Read the model definition and answer for the solid it produces. Units are mm, in the model's axes. Face numbers are marked on the shaded views. Give positions to 0.01 mm unless a question says otherwise; leave off trailing zeros. Write each loop counter-clockwise with the first axis right and the second up, starting at its lowest first coordinate (ties: lowest second). Pieces come first, ordered by that corner, then holes. Notation, with made-up numbers: M 74.25,31.5 L 120.25,31.5 A13 cw 120.25,56.5 Z; hole C 45,5 d4. An arc over 180 degrees is marked long. Put each result on its own line as item: value.
Autodesk Inventor part; units mm, degrees
ref_plane "YZ Plane" through (0, 0, 0) normal (1, 0, 0) x (0, 1, 0)
ref_plane "XZ Plane" through (0, 0, 0) normal (0, 1, 0) x (-1, 0, 0)
ref_plane "XY Plane" through (0, 0, 0) normal (0, 0, 1) x (1, 0, 0)
sketch "Sketch1" plane through (0, 0, 0) normal (0, 0, 1) x (1, 0, 0)
  circle A0 centre (-2.41, 40.64) radius 12.5
  line L0 (-16.506, 28.736) -> (-19.006, 26.236)
  arc A1 (-14.314, 26.544) -> (-16.506, 28.736) centre (-15.41, 27.64) ccw
  line L1 (-16.814, 24.044) -> (-14.314, 26.544)
  arc A2 (-19.006, 26.236) -> (-16.814, 24.044) centre (-17.91, 25.14) ccw
  line L2 (-19.006, 55.044) -> (-16.506, 52.544)
  arc A3 (-16.506, 52.544) -> (-14.314, 54.736) centre (-15.41, 53.64) ccw
  line L3 (-14.314, 54.736) -> (-16.814, 57.236)
  arc A4 (-16.814, 57.236) -> (-19.006, 55.044) centre (-17.91, 56.14) ccw
  line L4 (9.494, 26.544) -> (11.994, 24.044)
  arc A5 (11.686, 28.736) -> (9.494, 26.544) centre (10.59, 27.64) ccw
  line L5 (14.186, 26.236) -> (11.686, 28.736)
  arc A6 (11.994, 24.044) -> (14.186, 26.236) centre (13.09, 25.14) ccw
  line L6 (11.686, 52.544) -> (14.186, 55.044)
  arc A7 (9.494, 54.736) -> (11.686, 52.544) centre (10.59, 53.64) ccw
  line L7 (11.994, 57.236) -> (9.494, 54.736)
  arc A8 (14.186, 55.044) -> (11.994, 57.236) centre (13.09, 56.14) ccw
  circle A9 centre (20.14, 70.64) radius 2.5
  circle A10 centre (20.14, 10.64) radius 2.5
  circle A11 centre (100.14, 40.64) radius 3.57
  line L8 (-22.41, 20.64) -> (-22.41, 60.64)
  line L9 (-22.41, 60.64) -> (17.59, 80.64)
  line L10 (17.59, 80.64) -> (117.59, 80.64)
  line L11 (117.59, 80.64) -> (117.59, 0.64)
  line L12 (117.59, 0.64) -> (20.14, 0.64)
  line L13 (20.14, 0.64) -> (-22.41, 20.64)
  point P0 (0, 0)
  dimension "d0" = 20
  dimension "d1" = 0
  dimension "d2" = 80
  dimension "d3" = 90
  dimension "d4" = 90
  dimension "d5" = 10
  dimension "d6" = 100
  dimension "d7" = 140
  dimension "d8" = 40
  dimension "d9" = 20
extrude "Extrusion1" add sketch "Sketch1" along normal blind 3
fillet "Fillet1" radius 5 6 edges at (117.59, 80.64, 1.5) (117.59, 0.64, 1.5) (17.59, 80.64, 1.5) (-22.41, 60.64, 1.5) (-22.41, 20.64, 1.5) (20.14, 0.64, 1.5)
sketch "Sketch2" plane through (0, 0, 0) normal (0, 0, -1) x (-1, 0, 0)
  circle A0 centre (2.41, 40.64) radius 12.5
  circle A1 centre (-100.14, 40.64) radius 3.57
  circle A2 centre (-20.14, 10.64) radius 2.5
  circle A3 centre (-20.14, 70.64) radius 2.5
  arc A4 (-11.686, 52.544) -> (-9.494, 54.736) centre (-10.59, 53.64) ccw
  line L0 (-11.686, 52.544) -> (-14.186, 55.044)
  arc A5 (-11.994, 57.236) -> (-14.186, 55.044) centre (-13.09, 56.14) ccw
  line L1 (-11.994, 57.236) -> (-9.494, 54.736)
  arc A6 (-9.494, 26.544) -> (-11.686, 28.736) centre (-10.59, 27.64) ccw
  line L2 (-9.494, 26.544) -> (-11.994, 24.044)
  arc A7 (-14.186, 26.236) -> (-11.994, 24.044) centre (-13.09, 25.14) ccw
  line L3 (-14.186, 26.236) -> (-11.686, 28.736)
  arc A8 (19.006, 55.044) -> (16.814, 57.236) centre (17.91, 56.14) ccw
  line L4 (19.006, 55.044) -> (16.506, 52.544)
  arc A9 (14.314, 54.736) -> (16.506, 52.544) centre (15.41, 53.64) ccw
  line L5 (14.314, 54.736) -> (16.814, 57.236)
  arc A10 (16.506, 28.736) -> (14.314, 26.544) centre (15.41, 27.64) ccw
  line L6 (16.506, 28.736) -> (19.006, 26.236)
  arc A11 (16.814, 24.044) -> (19.006, 26.236) centre (17.91, 25.14) ccw
  line L7 (16.814, 24.044) -> (14.314, 26.544)
  arc A12 (-21.2565, 0.64) -> (-19.1296, 1.1149) centre (-21.2565, 5.64) ccw
  line L8 (-19.1296, 1.1149) -> (19.5369, 19.2896)
  arc A13 (19.5369, 19.2896) -> (22.41, 23.8146) centre (17.41, 23.8146) ccw
  line L9 (22.41, 23.8146) -> (22.41, 57.5498)
  arc A14 (22.41, 57.5498) -> (19.6461, 62.022) centre (17.41, 57.5498) ccw
  line L10 (19.6461, 62.022) -> (-16.5343, 80.1121)
  arc A15 (-16.5343, 80.1121) -> (-18.7703, 80.64) centre (-18.7703, 75.64) ccw
  line L11 (-18.7703, 80.64) -> (-112.59, 80.64)
  arc A16 (-112.59, 80.64) -> (-117.59, 75.64) centre (-112.59, 75.64) ccw
  line L12 (-117.59, 75.64) -> (-117.59, 5.64)
  arc A17 (-117.59, 5.64) -> (-112.59, 0.64) centre (-112.59, 5.64) ccw
  line L13 (-112.59, 0.64) -> (-21.2565, 0.64)
  point P0 (0, 0)
hole "Hole1" at (100.14, 40.64, 0) direction (0, 0, 1) diameter 12 depth 1
sketch "Sketch3" plane through (0, 0, 0) normal (0, 0, -1) x (-1, 0, 0)
  circle A0 centre (-20.14, 10.64) radius 2.5
  circle A1 centre (-100.14, 40.64) radius 6
  circle A2 centre (2.41, 40.64) radius 12.5
  circle A3 centre (-20.14, 10.64) radius 2.5
  circle A4 centre (-20.14, 70.64) radius 2.5
  arc A5 (-11.686, 52.544) -> (-9.494, 54.736) centre (-10.59, 53.64) ccw
  line L0 (-11.686, 52.544) -> (-14.186, 55.044)
  arc A6 (-11.994, 57.236) -> (-14.186, 55.044) centre (-13.09, 56.14) ccw
  line L1 (-11.994, 57.236) -> (-9.494, 54.736)
  arc A7 (-9.494, 26.544) -> (-11.686, 28.736) centre (-10.59, 27.64) ccw
  line L2 (-9.494, 26.544) -> (-11.994, 24.044)
  arc A8 (-14.186, 26.236) -> (-11.994, 24.044) centre (-13.09, 25.14) ccw
  line L3 (-14.186, 26.236) -> (-11.686, 28.736)
  arc A9 (19.006, 55.044) -> (16.814, 57.236) centre (17.91, 56.14) ccw
  line L4 (19.006, 55.044) -> (16.506, 52.544)
  arc A10 (14.314, 54.736) -> (16.506, 52.544) centre (15.41, 53.64) ccw
  line L5 (14.314, 54.736) -> (16.814, 57.236)
  arc A11 (16.506, 28.736) -> (14.314, 26.544) centre (15.41, 27.64) ccw
  line L6 (16.506, 28.736) -> (19.006, 26.236)
  arc A12 (16.814, 24.044) -> (19.006, 26.236) centre (17.91, 25.14) ccw
  line L7 (16.814, 24.044) -> (14.314, 26.544)
  arc A13 (-21.2565, 0.64) -> (-19.1296, 1.1149) centre (-21.2565, 5.64) ccw
  line L8 (-19.1296, 1.1149) -> (19.5369, 19.2896)
  arc A14 (19.5369, 19.2896) -> (22.41, 23.8146) centre (17.41, 23.8146) ccw
  line L9 (22.41, 23.8146) -> (22.41, 57.5498)
  arc A15 (22.41, 57.5498) -> (19.6461, 62.022) centre (17.41, 57.5498) ccw
  line L10 (19.6461, 62.022) -> (-16.5343, 80.1121)
  arc A16 (-16.5343, 80.1121) -> (-18.7703, 80.64) centre (-18.7703, 75.64) ccw
  line L11 (-18.7703, 80.64) -> (-112.59, 80.64)
  arc A17 (-112.59, 80.64) -> (-117.59, 75.64) centre (-112.59, 75.64) ccw
  line L12 (-117.59, 75.64) -> (-117.59, 5.64)
  arc A18 (-117.59, 5.64) -> (-112.59, 0.64) centre (-112.59, 5.64) ccw
  line L13 (-112.59, 0.64) -> (-21.2565, 0.64)
  circle A19 centre (-20.14, 70.64) radius 2.0572
  circle A20 centre (-20.14, 10.64) radius 2.0572
  point P0 (0, 0)
hole "Hole2" at (20.14, 10.64, 0) at (20.14, 70.64, 0) direction (0, 0, 1) diameter 8.1 depth 1
properties part number "Y Slider" material "Aluminum 6061"
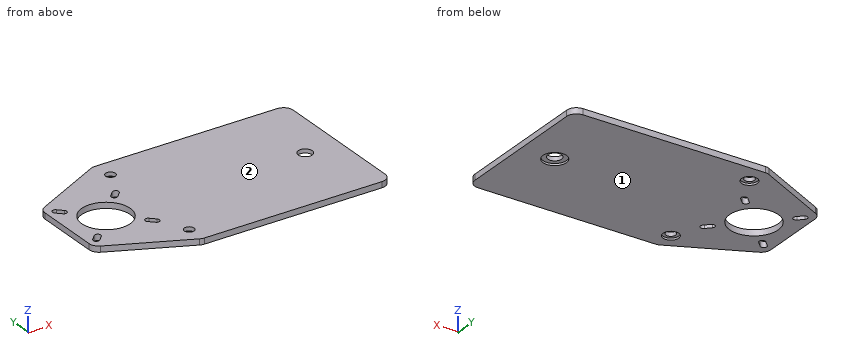
(1) Section B-B on z = 1.8 is taken. Give the number of separate pieces and of enclosed holes in the cut face, and give its area (3 significant figures).
Result:
separate pieces: 1
enclosed holes: 8
area: 9,720 mm²
(2) Section C-C on y = 40.64 is taken. Determine the outline of the cut face in (x, z).
Result:
outline: M -22.41,0 L -14.91,0 L -14.91,3 L -22.41,3 Z; M 10.09,0 L 94.14,0 L 94.14,1 L 96.57,1 L 96.57,3 L 10.09,3 Z; M 103.71,1 L 106.14,1 L 106.14,0 L 117.59,0 L 117.59,3 L 103.71,3 Z
(3) Straight lines are drawn through the part: line 1 along X through (y, z) = (56, 2.4); line 2 along X through (y, z) = (42.5, 2.1); line 3 along X through (y, z) = (7.5, 0.85). For each, find the intervals that lie inside material, in ascending order. Write a range as from..to.
Result:
line 1: x = -22.41..-19.45, -15.58..10.76, 14.63..117.59
line 2: x = -22.41..-14.77, 9.95..97.09, 103.19..117.59
line 3: x = 5.55..17.58, 22.7..117.59
(4) Section A-A on y = 70.64 is taken. Determine the outline of the cut face in (x, z), and give its area (3 significant figures).
Result:
outline: M -2.41,0 L 16.09,0 L 16.09,1 L 17.64,1 L 17.64,3 L -2.41,3 Z; M 22.64,1 L 24.19,1 L 24.19,0 L 117.59,0 L 117.59,3 L 22.64,3 Z
area: 342 mm²
(5) For a pull along Z with two mould halves and no side action, classify the marked faces 1 and 2 as +Z half, -Z half, draft (parallel to the pull), parting line (faces both ways), or undercut.
Result:
face 1: -Z half
face 2: +Z half
(6) Given pin 1 Ø10 at (x, y) = (-5.5, 44.5) entering from -Z; pin 2 Ø6.5 at (x, y) = (20.14, 70.64) entering from -Z, each flat-ended and moving along its own axis, determine where each tip first touches the part or whether it passes through.
Result:
pin 1: passes through
pin 2: stops at z = 1
(7) Section D-D on x = -5 is taken. Determine the outline of the cut face in (y, z) (3 decimals).
Result:
outline: M 12.457,0 L 28.411,0 L 28.411,3 L 12.457,3 Z; M 52.869,0 L 69.345,0 L 69.345,3 L 52.869,3 Z
